Geometry: final body of the model. Coordinates: model frame, mm. Give positions to 0.01 mm unless a question says otherwise; leave off trailing zeros. Write each loop counter-clockwise with the first axis right and the second up, starting at its lowest first coordinate (ties: lowest second). Pieces come first, ordered by that corner, then holes.
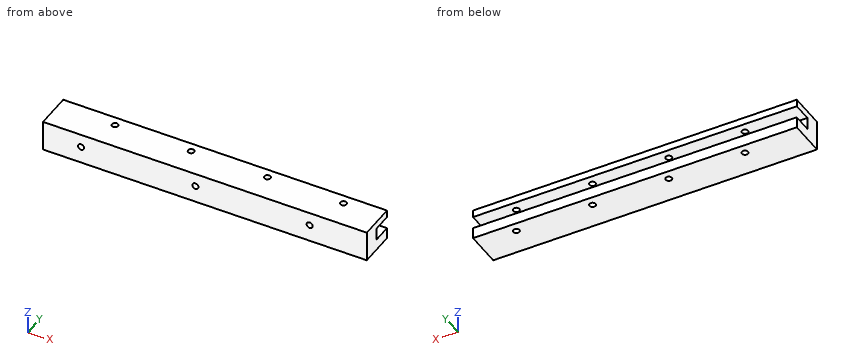
Autodesk Inventor part; units mm, degrees
ref_plane "YZ Plane" through (0, 0, 0) normal (1, 0, 0) x (0, 1, 0)
ref_plane "XZ Plane" through (0, 0, 0) normal (0, 1, 0) x (-1, 0, 0)
ref_plane "XY Plane" through (0, 0, 0) normal (0, 0, 1) x (1, 0, 0)
sketch "スケッチ1" plane through (0, 0, 0) normal (0, 1, 0) x (-1, 0, 0)
  line L0 (-90, -3) -> (90, -3)
  line L1 (90, -3) -> (90, 3)
  line L2 (90, 3) -> (-90, 3)
  line L3 (-90, 3) -> (-90, -3)
  line L4 (-90, -3) -> (90, 3) construction
  line L5 (90, -3) -> (-90, 3) construction
  point P0 (0, 0)
  dimension "d0" = 180
  dimension "d1" = 6
extrude "押し出し1" add sketch "スケッチ1" along normal blind 17
sketch "スケッチ2" plane through (0, 0, 0) normal (0, -1, 0) x (1, 0, 0)
  line L0 (-90, 3) -> (90, 3)
  line L1 (90, 3) -> (-80, 3)
  line L2 (-80, 3) -> (-80, 9)
  line L3 (-80, 9) -> (90, 9)
  line L4 (90, 9) -> (90, 3)
  line L5 (90, 3) -> (90, -3)
  line L6 (90, -3) -> (-80, -3)
  line L7 (-80, -3) -> (-80, -6)
  line L8 (-80, -6) -> (90, -6)
  line L9 (90, -6) -> (90, -3)
  point P0 (0, 0)
  dimension "d4" = 170
  dimension "d5" = 6
  dimension "d6" = 170
  dimension "d7" = 3
extrude "押し出し2" add sketch "スケッチ2" against normal blind 14
sketch "スケッチ3" plane through (0, 17, 0) normal (0, 1, 0) x (1, 0, 0)
  line L0 (-90, 3) -> (-90, -3)
  line L1 (90, -3) -> (90, 3)
  line L2 (-90, 3) -> (90, 3)
  line L3 (90, 3) -> (90, -3)
  line L4 (90, -3) -> (-90, -3)
  line L5 (-90, -3) -> (-90, 3)
  point P0 (0, 0)
extrude "押し出し3" cut sketch "スケッチ3" against normal blind 13
sketch "スケッチ4" plane through (0, 4, 0) normal (0, 1, 0) x (1, 0, 0)
  line L0 (-90, -3) -> (-90, 3)
  line L1 (-80, 6) -> (-80, 3)
  line L2 (-90, -3) -> (-80, -3)
  line L3 (-80, -3) -> (-80, 3)
  line L4 (-80, 3) -> (-90, 3)
  line L5 (-90, 3) -> (-90, -3)
  point P0 (0, 0)
extrude "押し出し4" cut sketch "スケッチ4" against normal blind 13
sketch "スケッチ5" plane through (0, 14, 0) normal (0, 1, 0) x (1, 0, 0)
  line L0 (97.0492, -3.2) -> (-97.0492, -3.2)
  line L1 (-97.0492, -3.2) -> (-97.0492, 3.2)
  line L2 (-97.0492, 3.2) -> (97.0492, 3.2)
  line L3 (97.0492, 3.2) -> (97.0492, -3.2)
  line L4 (97.0492, -3.2) -> (-97.0492, 3.2) construction
  line L5 (-97.0492, -3.2) -> (97.0492, 3.2) construction
  point P0 (0, 0)
  dimension "d14" = 6.4
extrude "押し出し5" cut sketch "スケッチ5" against normal blind 10
sketch "スケッチ6" plane through (-80, 0, 9) normal (0, 0, 1) x (1, 0, 0)
  line L0 (0, 14) -> (170, 14)
  line L1 (170, 0) -> (170, 14)
  point P0 (80, 0)
  point P1 (150, 9)
  point P2 (110, 9)
  point P3 (70, 9)
  point P4 (30, 9)
  dimension "d17" = 5
  dimension "d18" = 20
  dimension "d19" = 40
  dimension "d20" = 5
  dimension "d21" = 40
  dimension "d22" = 40
hole "穴1" at (70, 9, 9) at (30, 9, 9) at (-10, 9, 9) at (-50, 9, 9) direction (0, 0, -1) diameter 3.2 end through all
sketch "スケッチ7" plane through (0, 0, 0) normal (0, -1, 0) x (1, 0, 0)
  line L0 (-80, -6) -> (90, -6)
  line L1 (90, -6) -> (90, 9)
  line L2 (-80, -3.2) -> (90, -3.2)
  point P0 (0, 0)
  point P1 (60, 0)
  point P2 (0, 0)
  point P3 (-60, 0)
  dimension "d30" = 6
  dimension "d31" = 30
  dimension "d32" = 60
hole "穴2" at (60, 0, 0) at (0, 0, 0) at (-60, 0, 0) direction (0, 1, 0) diameter 3.2 end through all
sketch "スケッチ8" plane through (90, 0, -6) normal (0, 0, -1) x (-1, 0, 0)
  line L0 (170, 0) -> (170, 14)
  line L1 (0, 0) -> (170, 0)
  line L2 (170, 0) -> (170, 14)
  line L3 (170, 14) -> (0, 14)
  line L4 (0, 14) -> (0, 0)
  point P0 (90, 0)
extrude "押し出し6" add sketch "スケッチ8" along normal blind 3
sketch "スケッチ10" plane through (-80, 0, 9) normal (0, 0, 1) x (1, 0, 0)
  circle A0 centre (150, 9) radius 1.6
  circle A1 centre (110, 9) radius 1.6
  circle A2 centre (70, 9) radius 1.6
  circle A3 centre (30, 9) radius 1.6
  point P0 (80, 0)
hole "穴3" at (70, 9, 9) at (30, 9, 9) at (-10, 9, 9) at (-50, 9, 9) direction (0, 0, -1) diameter 3.2 end through all
sketch "スケッチ11" plane through (0, 14, 0) normal (0, 1, 0) x (1, 0, 0)
  line L0 (-80, -9) -> (90, -9)
  line L1 (-80, -9) -> (90, -9)
  line L2 (90, -9) -> (90, -6)
  line L3 (90, -6) -> (-80, -6)
  line L4 (-80, -6) -> (-80, -9)
  point P0 (0, 0)
  dimension "d49" = 170
  dimension "d50" = 3
extrude "押し出し7" cut sketch "スケッチ11" against normal blind 40
sketch "スケッチ12" plane through (-80, 14, 6) normal (0, 0, 1) x (1, 0, 0)
  line L0 (0, 0) -> (170, 0)
  line L1 (0, 0) -> (170, 0)
  line L2 (170, 0) -> (170, -14)
  line L3 (170, -14) -> (0, -14)
  line L4 (0, -14) -> (0, 0)
  point P0 (80, -14)
extrude "押し出し8" add sketch "スケッチ12" along normal blind 1
sketch "スケッチ13" plane through (0, 14, 0) normal (0, 1, 0) x (1, 0, 0)
  point P0 (0, 0)
sketch "スケッチ14" plane through (-80, 14, 7) normal (0, 0, 1) x (1, 0, 0)
  circle A0 centre (30, -5) radius 1.6
  circle A1 centre (70, -5) radius 1.6
  circle A2 centre (110, -5) radius 1.6
  circle A3 centre (150, -5) radius 1.6
  point P0 (80, -14)
hole "穴4" at (-50, 9, 7) at (-10, 9, 7) at (30, 9, 7) at (70, 9, 7) direction (0, 0, -1) diameter 3.2 depth 10
sketch "スケッチ15" plane through (0, 0, 0) normal (0, -1, 0) x (1, 0, 0)
  line L0 (-80, -9) -> (90, -9)
  line L1 (-80, 7) -> (90, 7)
  line L2 (90, 7) -> (90, -9)
  line L3 (90, -9) -> (-80, -9)
  line L4 (-80, -9) -> (-80, 7)
  point P0 (0, 0)
extrude "押し出し9" add sketch "スケッチ15" along normal blind 5
sketch "スケッチ16" plane through (0, -5, 0) normal (0, -1, 0) x (1, 0, 0)
  circle A0 centre (0, 0) radius 1.6
  circle A1 centre (-60, 0) radius 1.6
  circle A2 centre (60, 0) radius 1.6
hole "穴5" at (60, -5, 0) at (0, -5, 0) at (-60, -5, 0) direction (0, 1, 0) diameter 3.2 depth 10
properties part number "lock2"
Item 1: Section A-A, the plane z = 0. Return the cut outline in (x, y).
Found:
outline: (-80, -5) - (-61.6, -5) - (-61.6, 4) - (-80, 4) - close; (-58.4, -5) - (-1.6, -5) - (-1.6, 4) - (-58.4, 4) - close; (1.6, -5) - (58.4, -5) - (58.4, 4) - (1.6, 4) - close; (61.6, -5) - (90, -5) - (90, 4) - (61.6, 4) - close
Item 2: Section B-B, the plane x = 0. Return the cut outline in (y, z).
Found:
outline: (-5, -9) - (14, -9) - (14, -3.2) - (4, -3.2) - (4, -1.6) - (-5, -1.6) - close; (-5, 1.6) - (4, 1.6) - (4, 3.2) - (14, 3.2) - (14, 7) - (-5, 7) - close
Item 3: Section C-C, the plane x = -47. Return the cut outline in (y, z), plus the area to 3 significant figures.
Found:
outline: (-5, -9) - (14, -9) - (14, -3.2) - (4, -3.2) - (4, 3.2) - (14, 3.2) - (14, 7) - (-5, 7) - close
area: 240 mm2
Item 4: Line query: L1, parallel to X at y = 9, z = -5.4; L2, parallel to Z at x = -5.5, y = 6; L3, parallel to Y at x = 30, z = 4. Output: solid intervals per line, ascending.
Found:
L1: x = -80 to -51.6, -48.4 to -11.6, -8.4 to 28.4, 31.6 to 68.4, 71.6 to 90
L2: z = -9 to -3.2, 3.2 to 7
L3: y = -5 to 7.4, 10.6 to 14
Item 5: Pin query (flat end, axial travel): pin 1 Ø3 at (x, z) = (0, 0) entering from -Y. Return the tip coordinate at first contact, or that it passes through.
Found:
pin 1: passes through
